from build123d import *

# Parameters (mm, degrees)
F0_R     = 2.65
F0_R_2   = 4
F1_DEPTH = 6
F2_DEPTH = 4
F3_DEPTH = 2


with BuildPart() as f1:
    # F0 (on Right) → F1 (new body)
    with BuildSketch(Plane.YZ):
        with BuildLine():
            ThreePointArc((-2.2515407231, 36.53242851), (-2.6294191421, 36.8013801393), (-3.0879953604, 36.8709138028))
            ThreePointArc((-3.0879953604, 36.8709138028), (-18.5, 32.04293994), (-30.3871503338, 21.1097393303))
            ThreePointArc((-30.3871503338, 21.1097393303), (-30.5562205239, 20.6778338439), (-30.5122407901, 20.2161057189))
            ThreePointArc((-30.5122407901, 20.2161057189), (-30.7524645978, 17.7549437138), (-32.7637815132, 16.3163227911))
            ThreePointArc((-32.7637815132, 16.3163227911), (-33.185639666, 16.1235462954), (-33.4751456942, 15.7611744725))
            ThreePointArc((-33.4751456942, 15.7611744725), (-37, 0), (-33.4751456942, -15.7611744725))
            ThreePointArc((-33.4751456942, -15.7611744725), (-33.185639666, -16.1235462954), (-32.7637815132, -16.3163227911))
            ThreePointArc((-32.7637815132, -16.3163227911), (-30.7524645978, -17.7549437138), (-30.5122407901, -20.2161057189))
            ThreePointArc((-30.5122407901, -20.2161057189), (-30.5562205239, -20.6778338439), (-30.3871503338, -21.1097393303))
            ThreePointArc((-30.3871503338, -21.1097393303), (-18.5, -32.04293994), (-3.0879953604, -36.8709138028))
            ThreePointArc((-3.0879953604, -36.8709138028), (-2.6294191421, -36.8013801393), (-2.2515407231, -36.53242851))
            ThreePointArc((-2.2515407231, -36.53242851), (0, -35.5098874275), (2.2515407231, -36.53242851))
            ThreePointArc((2.2515407231, -36.53242851), (2.6294191421, -36.8013801393), (3.0879953604, -36.8709138028))
            ThreePointArc((3.0879953604, -36.8709138028), (18.5, -32.04293994), (30.3871503338, -21.1097393303))
            ThreePointArc((30.3871503338, -21.1097393303), (30.5562205239, -20.6778338439), (30.5122407901, -20.2161057189))
            ThreePointArc((30.5122407901, -20.2161057189), (30.7524645978, -17.7549437138), (32.7637815132, -16.3163227911))
            ThreePointArc((32.7637815132, -16.3163227911), (33.185639666, -16.1235462954), (33.4751456942, -15.7611744725))
            ThreePointArc((33.4751456942, -15.7611744725), (37, 0), (33.4751456942, 15.7611744725))
            ThreePointArc((33.4751456942, 15.7611744725), (33.185639666, 16.1235462954), (32.7637815132, 16.3163227911))
            ThreePointArc((32.7637815132, 16.3163227911), (31.941237039, 16.6082774884), (31.2380455813, 17.1253255822))
            ThreePointArc((31.2380455813, 17.1253255822), (29.4448637287, 17), (30.449989793, 18.4902782469))
            ThreePointArc((30.449989793, 18.4902782469), (30.3538087376, 19.3577839598), (30.5122407901, 20.2161057189))
            ThreePointArc((30.5122407901, 20.2161057189), (30.5562205239, 20.6778338439), (30.3871503338, 21.1097393303))
            ThreePointArc((30.3871503338, 21.1097393303), (18.5, 32.04293994), (3.0879953604, 36.8709138028))
            ThreePointArc((3.0879953604, 36.8709138028), (2.6294191421, 36.8013801393), (2.2515407231, 36.53242851))
            ThreePointArc((2.2515407231, 36.53242851), (0, 35.5098874275), (-2.2515407231, 36.53242851))
        make_face()
        with BuildLine():
            Line((-23.0952370323, 14.180454946), (-17.0328632471, 23.8484731203))
            ThreePointArc((-17.0328632471, 23.8484731203), (0.0002590164, 33.2703478915), (17.0295377344, 23.8415279974))
            Line((17.0295377344, 23.8415279974), (23.0899184639, 14.167925942))
            ThreePointArc((23.0899184639, 14.167925942), (23.4636524397, 13.5467460522), (23.8147430167, 12.9124929901))
            Line((23.8147430167, 12.9124929901), (29.162137778, 2.827248294))
            ThreePointArc((29.162137778, 2.827248294), (28.813095975, -16.6349496309), (12.1369519401, -26.6751288313))
            Line((12.1369519401, -26.6751288313), (0.7330157043, -27.0912894495))
            ThreePointArc((0.7330157043, -27.0912894495), (0, -27.1046598669), (-0.7330157043, -27.0912894495))
            Line((-0.7330157043, -27.0912894495), (-12.1441739659, -26.6748652799))
            ThreePointArc((-12.1441739659, -26.6748652799), (-28.8182692269, -16.6382354957), (-29.1731979579, 2.8202694775))
            Line((-29.1731979579, 2.8202694775), (-23.8282527367, 12.9108345034))
            ThreePointArc((-23.8282527367, 12.9108345034), (-23.4733240056, 13.5523299334), (-23.0952370323, 14.180454946))
        make_face(mode=Mode.SUBTRACT)
        with BuildLine():
            ThreePointArc((17.0295377344, 23.8415279974), (0.0002590164, 33.2703478915), (-17.0328632471, 23.8484731203))
            Line((-17.0328632471, 23.8484731203), (-23.0952370323, 14.180454946))
            ThreePointArc((-23.0952370323, 14.180454946), (-23.4733240056, 13.5523299334), (-23.8282527367, 12.9108345034))
            Line((-23.8282527367, 12.9108345034), (-29.1731979579, 2.8202694775))
            ThreePointArc((-29.1731979579, 2.8202694775), (-28.8182692269, -16.6382354957), (-12.1441739659, -26.6748652799))
            Line((-12.1441739659, -26.6748652799), (-0.7330157043, -27.0912894495))
            ThreePointArc((-0.7330157043, -27.0912894495), (0, -27.1046598669), (0.7330157043, -27.0912894495))
            Line((0.7330157043, -27.0912894495), (12.1369519401, -26.6751288313))
            ThreePointArc((12.1369519401, -26.6751288313), (28.813095975, -16.6349496309), (29.162137778, 2.827248294))
            Line((29.162137778, 2.827248294), (23.8147430167, 12.9124929901))
            ThreePointArc((23.8147430167, 12.9124929901), (23.4636524397, 13.5467460522), (23.0899184639, 14.167925942))
            Line((23.0899184639, 14.167925942), (17.0295377344, 23.8415279974))
        make_face()
        with BuildLine():
            Line((-14.5383641102, 8.8148297318), (-8.4759903249, 18.482847906))
            ThreePointArc((-8.4759903249, 18.482847906), (-0.0018003141, 23.1703476982), (8.4704774851, 18.4793926211))
            Line((8.4704774851, 18.4793926211), (14.5308582146, 8.8057905657))
            ThreePointArc((14.5308582146, 8.8057905657), (14.7167955123, 8.4967458506), (14.8914674376, 8.1811970698))
            Line((14.8914674376, 8.1811970698), (20.2388621989, -1.9040476263))
            ThreePointArc((20.2388621989, -1.9040476263), (20.0652095641, -11.5867329668), (11.7686206585, -16.5818468966))
            Line((11.7686206585, -16.5818468966), (0.3646844227, -16.9980075148))
            ThreePointArc((0.3646844227, -16.9980075148), (0, -17.0046594636), (-0.3646844227, -16.9980075148))
            Line((-0.3646844227, -16.9980075148), (-11.7758426843, -16.5815833453))
            ThreePointArc((-11.7758426843, -16.5815833453), (-20.0714122995, -11.5882352941), (-20.2479937541, -1.9073872429))
            Line((-20.2479937541, -1.9073872429), (-14.9030485329, 8.183177783))
            ThreePointArc((-14.9030485329, 8.183177783), (-14.7264670782, 8.5023297318), (-14.5383641102, 8.8148297318))
        make_face(mode=Mode.SUBTRACT)
        with BuildLine():
            ThreePointArc((8.4704774851, 18.4793926211), (-0.0018003141, 23.1703476982), (-8.4759903249, 18.482847906))
            Line((-8.4759903249, 18.482847906), (-14.5383641102, 8.8148297318))
            ThreePointArc((-14.5383641102, 8.8148297318), (-14.7264670782, 8.5023297318), (-14.9030485329, 8.183177783))
            Line((-14.9030485329, 8.183177783), (-20.2479937541, -1.9073872429))
            ThreePointArc((-20.2479937541, -1.9073872429), (-20.0714122995, -11.5882352941), (-11.7758426843, -16.5815833453))
            Line((-11.7758426843, -16.5815833453), (-0.3646844227, -16.9980075148))
            ThreePointArc((-0.3646844227, -16.9980075148), (0, -17.0046594636), (0.3646844227, -16.9980075148))
            Line((0.3646844227, -16.9980075148), (11.7686206585, -16.5818468966))
            ThreePointArc((11.7686206585, -16.5818468966), (20.0652095641, -11.5867329668), (20.2388621989, -1.9040476263))
            Line((20.2388621989, -1.9040476263), (14.8914674376, 8.1811970698))
            ThreePointArc((14.8914674376, 8.1811970698), (14.7167955123, 8.4967458506), (14.5308582146, 8.8057905657))
            Line((14.5308582146, 8.8057905657), (8.4704774851, 18.4793926211))
        make_face()
        with Locations((-12.5573683549, -7.25)):
            Circle(F0_R, mode=Mode.SUBTRACT)
        with Locations((12.5573683549, -7.25)):
            Circle(F0_R, mode=Mode.SUBTRACT)
        Circle(F0_R_2, mode=Mode.SUBTRACT)
        with Locations((0, 14.5)):
            Circle(F0_R, mode=Mode.SUBTRACT)
    extrude(amount=-F1_DEPTH)

    # F0 (on Right) → F2 (cut)
    with BuildSketch(Plane.YZ):
        with BuildLine():
            ThreePointArc((17.0295377344, 23.8415279974), (0.0002590164, 33.2703478915), (-17.0328632471, 23.8484731203))
            Line((-17.0328632471, 23.8484731203), (-23.0952370323, 14.180454946))
            ThreePointArc((-23.0952370323, 14.180454946), (-23.4733240056, 13.5523299334), (-23.8282527367, 12.9108345034))
            Line((-23.8282527367, 12.9108345034), (-29.1731979579, 2.8202694775))
            ThreePointArc((-29.1731979579, 2.8202694775), (-28.8182692269, -16.6382354957), (-12.1441739659, -26.6748652799))
            Line((-12.1441739659, -26.6748652799), (-0.7330157043, -27.0912894495))
            ThreePointArc((-0.7330157043, -27.0912894495), (0, -27.1046598669), (0.7330157043, -27.0912894495))
            Line((0.7330157043, -27.0912894495), (12.1369519401, -26.6751288313))
            ThreePointArc((12.1369519401, -26.6751288313), (28.813095975, -16.6349496309), (29.162137778, 2.827248294))
            Line((29.162137778, 2.827248294), (23.8147430167, 12.9124929901))
            ThreePointArc((23.8147430167, 12.9124929901), (23.4636524397, 13.5467460522), (23.0899184639, 14.167925942))
            Line((23.0899184639, 14.167925942), (17.0295377344, 23.8415279974))
        make_face()
        with BuildLine():
            Line((-14.5383641102, 8.8148297318), (-8.4759903249, 18.482847906))
            ThreePointArc((-8.4759903249, 18.482847906), (-0.0018003141, 23.1703476982), (8.4704774851, 18.4793926211))
            Line((8.4704774851, 18.4793926211), (14.5308582146, 8.8057905657))
            ThreePointArc((14.5308582146, 8.8057905657), (14.7167955123, 8.4967458506), (14.8914674376, 8.1811970698))
            Line((14.8914674376, 8.1811970698), (20.2388621989, -1.9040476263))
            ThreePointArc((20.2388621989, -1.9040476263), (20.0652095641, -11.5867329668), (11.7686206585, -16.5818468966))
            Line((11.7686206585, -16.5818468966), (0.3646844227, -16.9980075148))
            ThreePointArc((0.3646844227, -16.9980075148), (0, -17.0046594636), (-0.3646844227, -16.9980075148))
            Line((-0.3646844227, -16.9980075148), (-11.7758426843, -16.5815833453))
            ThreePointArc((-11.7758426843, -16.5815833453), (-20.0714122995, -11.5882352941), (-20.2479937541, -1.9073872429))
            Line((-20.2479937541, -1.9073872429), (-14.9030485329, 8.183177783))
            ThreePointArc((-14.9030485329, 8.183177783), (-14.7264670782, 8.5023297318), (-14.5383641102, 8.8148297318))
        make_face(mode=Mode.SUBTRACT)
    extrude(amount=-F2_DEPTH, mode=Mode.SUBTRACT)

    # F3 (add): a face of the model
    f3_faces = [f1.faces().sort_by_distance(p)[0] for p in [
        (0, -11.0097556238, 13.3369283968),
    ]]
    extrude(f3_faces, amount=F3_DEPTH)


solid = f1.part
For this review, take the finished solid that the model builds, in its own axes (mm). A direction names the side the tool comes from. Give positions to 0.01 mm unless a question says otherwise; leave off trailing zeros. Order: outer loops, then holes, each group sorted by start corner. A loop starts at its lowest first (then second) coordinate and runs counter-clockwise, first axis right, second up. Notation, with made-up numbers: M 11,-4 L 68,-4 A27 ccw 68,30 Z; hole C 48,53 d11. An arc over 180 degrees is marked long. Answer in a Markdown table with one row per item. Add a question column.
(1) Mouldability with a two-part tool opening along Z and no side actions: class faces 3 (the face through (-2.06, -14.66, -8.86)), 4 (the face through (-2.958, 18.302, -32.156)), 5 (the face through (0, -22, 17)) as +Z half, -Z half, draft (parallel to the pull), parting line (faces both ways), or undercut.
(2) For pin 1 (5 mm diameter, centred on y = -29, z = -23, fed in from +X); pin 2 (1.6 mm diameter, centred on y = 30.31, z = 17.5, fed in from +X); pin 3 (1 mm diameter, centred on x = 0, y = -1, fed in from +Z); pin 4 (1.5 mm diameter, centred on x = 0.5, z = 1.5, fed in from -Y), all flat-tipped, find the tip position at first contact; note any pin that passes through.
(3) Consider section B-B on x = -2.5. Give the number of separate pieces and of enclosed holes in the cut face, and give its area (3 significant figures).
(4) Consider section C-C on y = -28. State the section outline as (x, z) points, and give its area (3 significant figures).
(5) Wall thickness on probe 1 along Z at (x, y) = (-3.5, 0); probe 2 along Z at (x, y) = (0.5, 0); probe 3 along Y at (x, z) = (-2.75, 22): over which ranges is each line inside the solid? List them lowest first. Write a range as [from, to].
(6) For faces 1 (the face through (-2.056, -0.867, -3.905)), 2 (the face through (-1.97, 0.28, 33.27)), list the 3-axis set-ups (+Z, -Z, +X, -X, +Y, -Y) from which the entire face can be reached by the end or side of a thin tool; tool diameter is ignored.
(7) Consider section D-D on z = -24. State the section outline as (x, y) points, and give its area (3 significant figures).
(8) Consider section A-A on z = 0. State the section outline as (x, y) points.
Evaluation:
| question | item | result |
|---|---|---|
| 1 | face 3 | undercut |
| 1 | face 4 | -Z half |
| 1 | face 5 | draft |
| 2 | pin 1 | stops at x = 0 |
| 2 | pin 2 | passes through |
| 2 | pin 3 | stops at z = 35.91 |
| 2 | pin 4 | stops at y = -36.99 |
| 3 | separate pieces | 2 |
| 3 | enclosed holes | 5 |
| 3 | area | 2,500 mm^2 |
| 4 | outline | M -6,-24.19 L 0,-24.19 L 0,-17.94 L -4,-17.94 L -4,5.04 L 0,5.04 L 0,24.19 L -6,24.19 Z |
| 4 | area | 198 mm^2 |
| 5 | probe 1 | z = [-35.51, -27.1], [-17, -4], [4, 11.85], [17.15, 23.17], [33.27, 35.51] |
| 5 | probe 2 | z = [-17, -4], [4, 11.85], [17.15, 23.17] |
| 5 | probe 3 | y = [-29.75, -18.19], [-4.7, 4.69], [18.18, 29.75] |
| 6 | face 1 | +X, -X |
| 6 | face 2 | +X |
| 7 | outline | M -6,-28.16 L 0,-28.16 L 0,-21.45 L -4,-21.45 L -4,21.45 L 0,21.45 L 0,28.16 L -6,28.16 Z |
| 7 | area | 166 mm^2 |
| 8 | outline | M -6,-37 L 0,-37 L 0,-30.4 L -4,-30.4 L -4,-19.24 L 2,-19.24 L 2,-4 L -6,-4 Z; M -6,4 L 2,4 L 2,19.23 L -4,19.23 L -4,30.39 L 0,30.39 L 0,37 L -6,37 Z |
